from build123d import *

# Parameters (mm, degrees)
SKETCH_W        = 88
SKETCH_H        = 58
PAD_DEPTH       = 2
SKETCH001_W     = 1
SKETCH001_H     = 11
PAD001_DEPTH    = 8
SKETCH002_W     = 1
SKETCH002_H     = 11
PAD002_DEPTH    = 8
SKETCH003_W     = 26
SKETCH003_H     = 1
PAD003_DEPTH    = 8
SKETCH004_W     = 15
SKETCH004_H     = 19
PAD004_DEPTH    = 3
SKETCH005_W     = 28
SKETCH005_H     = 10
PAD005_DEPTH    = 3
SKETCH006_R     = 1.5
PAD006_DEPTH    = 22
PAD007_DEPTH    = 22
SKETCH007_W     = 8
SKETCH007_H     = 5
PAD008_DEPTH    = 3
SKETCH008_R     = 2.5
PAD009_DEPTH    = 1
SKETCH009_R     = 1.5
PAD010_DEPTH    = 15
SKETCH010_W     = 2
SKETCH010_H     = 58
SKETCH010_W_2   = 1
PAD011_DEPTH    = 38
SKETCH011_W     = 85
SKETCH011_H     = 2
SKETCH011_H_2   = 1.5
PAD012_DEPTH    = 38
SKETCH012_R     = 0.75
SKETCH012_R_2   = 0.6
PAD013_DEPTH    = 2
POCKET_DEPTH    = 1.5
SKETCH014_W     = 21
SKETCH014_H     = 15
POCKET001_DEPTH = 1.5


with BuildPart() as part:
    # Sketch → Pad (new body)
    with BuildSketch(Plane.XY):
        with Locations((44, 29)):
            Rectangle(SKETCH_W, SKETCH_H)
    extrude(amount=PAD_DEPTH)

    # Sketch001 (on Face6 of Pad) → Pad001 (join)
    with BuildSketch(Plane.XY.offset(2)):
        with Locations((5.5, 17.5)):
            Rectangle(SKETCH001_W, SKETCH001_H)
    extrude(amount=PAD001_DEPTH)

    # Sketch002 (on Face5 of Pad001) → Pad002 (join)
    with BuildSketch(Plane.XY.offset(2)):
        with Locations((82.5, 17.5)):
            Rectangle(SKETCH002_W, SKETCH002_H)
    extrude(amount=PAD002_DEPTH)

    # Sketch003 (on Face5 of Pad002) → Pad003 (join)
    with BuildSketch(Plane.XY.offset(2)):
        with Locations((43, 6.5)):
            Rectangle(SKETCH003_W, SKETCH003_H)
        with Locations((43, 28.5)):
            Rectangle(SKETCH003_W, SKETCH003_H)
    extrude(amount=PAD003_DEPTH)

    # Sketch004 (on Face5 of Pad003) → Pad004 (join)
    with BuildSketch(Plane.XY.offset(2)):
        with Locations((10.5, 45.5)):
            Rectangle(SKETCH004_W, SKETCH004_H)
    extrude(amount=PAD004_DEPTH)

    # Sketch005 (on Face5 of Pad004) → Pad005 (join)
    with BuildSketch(Plane.XY.offset(2)):
        with Locations((60, 41)):
            Rectangle(SKETCH005_W, SKETCH005_H)
    extrude(amount=PAD005_DEPTH)

    # Sketch006 (on Face5 of Pad005) → Pad006 (join)
    with BuildSketch(Plane.XY.offset(2)):
        with Locations((84, 5)):
            Circle(SKETCH006_R)
        with Locations((20.5, 5)):
            Circle(SKETCH006_R)
        with Locations((20.5, 45.5)):
            Circle(SKETCH006_R)
        with Locations((84, 45.5)):
            Circle(SKETCH006_R)
    extrude(amount=PAD006_DEPTH)

    # Sketch006 (on Face5 of Pad005) → Pad007 (join)
    with BuildSketch(Plane.XY.offset(2)):
        with Locations((84, 5)):
            Circle(SKETCH006_R)
        with Locations((20.5, 5)):
            Circle(SKETCH006_R)
        with Locations((20.5, 45.5)):
            Circle(SKETCH006_R)
        with Locations((84, 45.5)):
            Circle(SKETCH006_R)
    extrude(amount=PAD007_DEPTH)

    # Sketch007 (on Face5 of Pad007) → Pad008 (join)
    with BuildSketch(Plane.XY.offset(2)):
        with Locations((29.5, 51.5)):
            Rectangle(SKETCH007_W, SKETCH007_H)
    extrude(amount=PAD008_DEPTH)

    # Sketch008 (on Face35 of Pad007) → Pad009 (join)
    with BuildSketch(Plane.XY.offset(24)):
        with Locations((20.5, 5)):
            Circle(SKETCH008_R)
        with Locations((84, 5)):
            Circle(SKETCH008_R)
        with Locations((20.5, 45.5)):
            Circle(SKETCH008_R)
        with Locations((84, 45.5)):
            Circle(SKETCH008_R)
    extrude(amount=PAD009_DEPTH)

    # Sketch009 (on Face54 of Pad009) → Pad010 (join)
    with BuildSketch(Plane.XY.offset(25)):
        with Locations((20.5, 5)):
            Circle(SKETCH009_R)
        with Locations((84, 5)):
            Circle(SKETCH009_R)
        with Locations((20.5, 45.5)):
            Circle(SKETCH009_R)
        with Locations((84, 45.5)):
            Circle(SKETCH009_R)
    extrude(amount=PAD010_DEPTH)

    # Sketch010 (on Face5 of Pad010) → Pad011 (join)
    with BuildSketch(Plane.XY.offset(2)):
        with Locations((1, 29)):
            Rectangle(SKETCH010_W, SKETCH010_H)
        with Locations((87.5, 29.00001)):
            Rectangle(SKETCH010_W_2, SKETCH010_H)
    extrude(amount=PAD011_DEPTH)

    # Sketch011 (on Face5 of Pad010) → Pad012 (join)
    with BuildSketch(Plane.XY.offset(2)):
        with Locations((44.5, 1)):
            Rectangle(SKETCH011_W, SKETCH011_H)
        with Locations((44.5, 57.25)):
            Rectangle(SKETCH011_W, SKETCH011_H_2)
    extrude(amount=PAD012_DEPTH)

    # Sketch012 (on Face11 of Pad012) → Pad013 (join)
    with BuildSketch(Plane.XY.offset(40)):
        with Locations((1.5, 1.2)):
            Circle(SKETCH012_R)
        with Locations((1.2, 57)):
            Circle(SKETCH012_R)
        with Locations((87.2, 57.2)):
            Circle(SKETCH012_R_2)
        with Locations((87, 1)):
            Circle(SKETCH012_R)
    extrude(amount=PAD013_DEPTH)

    # Sketch013 (on Face15 of Pad013) → Pocket (cut)
    with BuildSketch(Plane(origin=(0, 58, 0), x_dir=(-1, 0, 0), z_dir=(0, 1, 0))):
        with BuildLine():
            ThreePointArc((-8, 5), (-7, 6), (-8, 7))
            Line((-8, 7), (-13.5, 7))
            ThreePointArc((-13.5, 7), (-14.5, 6), (-13.5, 5))
            Line((-8, 5), (-13.5, 5))
        make_face()
    extrude(amount=-POCKET_DEPTH, mode=Mode.SUBTRACT)

    # Sketch014 (on Face15 of Pocket) → Pocket001 (cut)
    with BuildSketch(Plane(origin=(0, 58, 0), x_dir=(-1, 0, 0), z_dir=(0, 1, 0))):
        with Locations((-30.5, 11.5)):
            Rectangle(SKETCH014_W, SKETCH014_H)
    extrude(amount=-POCKET001_DEPTH, mode=Mode.SUBTRACT)


solid = part.part
Could you check a few things on this model? Use its own coordinates, in mm. A direction names the side the tool comes from. Coordinates: 2 decimals unless noted, no trailing zeros. Order: outer loops, then holes, each group sorted by start corner. A loop starts at its lowest first (then second) coordinate and runs counter-clockwise, first axis right, second up. Notation, with made-up numbers: (81, 63.5) -> (89, 63.5) arc R30 cw to (89, 93.5) -> close; hole circle Ø10 at (58.5, 83). An arc over 180 degrees is marked (long way). One line per item, written item: value. Start each with the question number.
1) Which directions (+Z, -Z, +X, -X, +Y, -Y) give clear straight access to the entire face, cutting with the end or side of a thin tool? Please do faces 3 (the flat face through (25.5, 51, 3)), 4 (the flat face through (84, 46, 40)), 5 (the cylindrical face through (85.43, 5.45, 12.85)).
2) Imagine slicing it at C-C on y = 25.5. List the corners of the cut face in (x, z) for me, plus the area to 3 significant figures.
3) We'd pull the mould along Y, two halves only. Please class faces 1 (the flat face through (29, 49, 3)), 2 (the flat face through (20, 5, 40)): +Y half, -Y half, draft (parallel to the pull), parting line (faces both ways), or undercut.
4) Imagine slicing it at A-A on z = 37.5. Count the separate pieces of the cut face and the enclosed holes in it, plus the area to 3 significant figures.
5) If I drill on L1, parallel to X at y = 43, z = 4; L2, parallel to Y at x = 66, z = 3; L3, parallel to Y at x = 48.5, z = 16.5, over which ranges is the centre line in solid material (lowest first)? Write a range as [from, to].
6) I'm going to push flat-ended pins straight in: pin 1 (1.5 mm diameter, centred on y = 42.5, z = 4, fed in from -X); pin 2 (0.8 mm diameter, centred on x = 82.5, y = 16.5, fed in from +Z); pin 3 (6 mm diameter, centred on x = 41.5, y = 11, fed in from +Z). Where does each tip first touch, or does it pass through?
Answer list:
1. face 3: +Z
1. face 4: +Z, +X, -X, +Y, -Y
1. face 5: none
2. outline: (0, 0) -> (88, 0) -> (88, 40) -> (87, 40) -> (87, 2) -> (2, 2) -> (2, 40) -> (0, 40) -> close
2. area: 290 mm2
3. face 1: undercut
3. face 2: draft
4. separate pieces: 5
4. enclosed holes: 1
4. area: 500 mm2
5. L1: x = [0, 2], [3, 18], [46, 74], [87, 88]
5. L2: y = [0, 2], [36, 46], [56.5, 58]
5. L3: y = [0, 2], [56.5, 58]
6. pin 1: stops at x = 0
6. pin 2: stops at z = 10
6. pin 3: stops at z = 2
